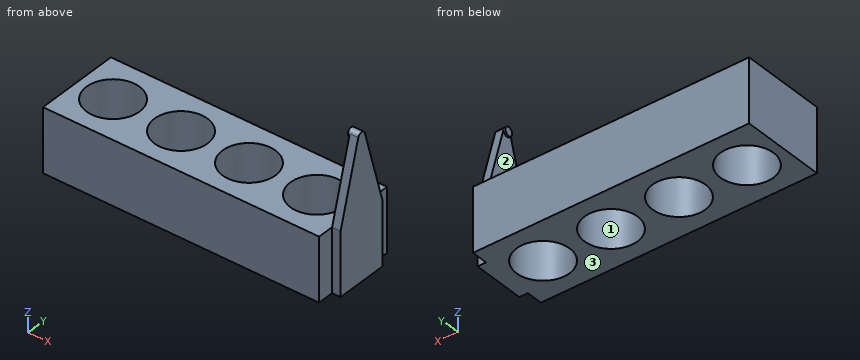
```python
from build123d import *

# Parameters (mm, degrees)
F0_W     = 130
F0_H     = 40
F0_R     = 12.5
F1_DEPTH = 30
F2_W     = 12.3288280059
F2_H     = 30
F3_DEPTH = 4
F4_DEPTH = 4
F6_DEPTH = 0.88206


with BuildPart() as f1:
    # F0 (on Top) → F1 (new body)
    with BuildSketch(Plane.XY):
        Rectangle(F0_W, F0_H)
        with Locations((-48, 0)):
            Circle(F0_R, mode=Mode.SUBTRACT)
        with Locations((-16, 0)):
            Circle(F0_R, mode=Mode.SUBTRACT)
        with Locations((16, 0)):
            Circle(F0_R, mode=Mode.SUBTRACT)
        with Locations((48, 0)):
            Circle(F0_R, mode=Mode.SUBTRACT)
    extrude(amount=F1_DEPTH)

    # F2 (on face) → F3 (join)
    with BuildSketch(Plane.YZ.offset(65)):
        with BuildLine():
            Line((-12.3288280059, 30), (0, 30))
            Line((0, 30), (0, 64))
            ThreePointArc((0, 64), (-1.5961346024, 64.7948633558), (-1.9235602984, 66.5476456688))
            Line((-1.9235602984, 66.5476456688), (-12.3288280059, 30))
        make_face()
        with BuildLine():
            Line((0, 64), (0, 30))
            Line((0, 30), (12.3288280059, 30))
            Line((12.3288280059, 30), (1.9235602984, 66.5476456688))
            ThreePointArc((1.9235602984, 66.5476456688), (1.9807978944, 66.2764773076), (2, 66))
            ThreePointArc((2, 66), (1.4142135624, 64.5857864376), (0, 64))
        make_face()
        with Locations((6.164414003, 15)):
            Rectangle(F2_W, F2_H)
        with Locations((-6.164414003, 15)):
            Rectangle(F2_W, F2_H)
    extrude(amount=F3_DEPTH)

    # F2 (on face) → F4 (join)
    with BuildSketch(Plane.YZ.offset(65)):
        with BuildLine():
            Line((0, 0), (0, 30))
            Line((0, 30), (0, 64))
            ThreePointArc((0, 64), (-1.5961346024, 64.7948633558), (-1.9235602984, 66.5476456688))
            Line((-1.9235602984, 66.5476456688), (-12.3288280059, 30))
            Line((-12.3288280059, 30), (-12.3288280059, 0))
            Line((-12.3288280059, 0), (0, 0))
        make_face()
        with BuildLine():
            Line((0, 64), (0, 30))
            Line((0, 30), (0, 0))
            Line((0, 0), (12.3288280059, 0))
            Line((12.3288280059, 0), (12.3288280059, 30))
            Line((12.3288280059, 30), (1.9235602984, 66.5476456688))
            ThreePointArc((1.9235602984, 66.5476456688), (1.9807978944, 66.2764773076), (2, 66))
            ThreePointArc((2, 66), (1.4142135624, 64.5857864376), (0, 64))
        make_face()
        with BuildLine():
            ThreePointArc((-1.9235602984, 66.5476456688), (-1.5961346024, 64.7948633558), (0, 64))
            ThreePointArc((0, 64), (1.4142135624, 64.5857864376), (2, 66))
            ThreePointArc((2, 66), (1.9807978944, 66.2764773076), (1.9235602984, 66.5476456688))
            ThreePointArc((1.9235602984, 66.5476456688), (0, 68), (-1.9235602984, 66.5476456688))
        make_face()
    extrude(amount=F4_DEPTH)

    # F5 (on face) → F6 (join)
    with BuildSketch(Plane(origin=(65, 0, 0), x_dir=(0, -1, 0), z_dir=(-1, 0, 0))):
        with BuildLine():
            ThreePointArc((-1.9235602984, 66.5476456688), (-0.2764773076, 64.0192021056), (2, 66))
            ThreePointArc((2, 66), (1.9807978944, 66.2764773076), (1.9235602984, 66.5476456688))
            ThreePointArc((1.9235602984, 66.5476456688), (0, 68), (-1.9235602984, 66.5476456688))
        make_face()
    extrude(amount=F6_DEPTH)


solid = f1.part
```
Build history of the part. All positions in model axes, mm. Face numbers are marked on the shaded views. Give positions to 0.01 mm unless a question says otherwise; leave off trailing zeros. Loops run counter-clockwise (first coordinate to the right, second up) from the corner with the lowest first, then second, coordinate; pieces in that order, holes last.
Item 1: Pull direction Z, two halves, no side cores. Call the marked faces 1, 2 and 3: released by +Z, released by -Z, zero draft, split by the parting line, or undercut.
Answers follow:
face 1: zero draft
face 2: undercut
face 3: released by -Z
Item 2: Slice it at C-C, the plane z = 22.5. List the corners of the cut face in (x, y).
Answers follow:
outline: (-65, -20) - (65, -20) - (65, -12.33) - (69, -12.33) - (69, 12.33) - (65, 12.33) - (65, 20) - (-65, 20) - close; hole circle Ø25 at (-48, 0); hole circle Ø25 at (-16, 0); hole circle Ø25 at (16, 0); hole circle Ø25 at (48, 0)
Item 3: Slice it at B-B, the plane x = 58. List the corners of the cut face in (y, z), and give its area (3 significant figures).
Answers follow:
outline: (-20, 0) - (-7.5, 0) - (-7.5, 30) - (-20, 30) - close; (7.5, 0) - (20, 0) - (20, 30) - (7.5, 30) - close
area: 750 mm2
Item 4: Drill centre lines: line 1 (Y direction, x = -48, z = 14); line 2 (Z direction, x = -21, y = -12.5); line 3 (Y direction, x = -37.5, z = 15.5). Where is each one in solid material? Low to high.
Answers follow:
line 1: y = -20 to -12.5, 12.5 to 20
line 2: z = 0 to 30
line 3: y = -20 to -6.78, 6.78 to 20
Item 5: Slice it at A-A, the plane y = 0. List the corners of the cut face in (x, z), and give its area (3 significant figures).
Answers follow:
outline: (-65, 0) - (-60.5, 0) - (-60.5, 30) - (-65, 30) - close; (-35.5, 0) - (-28.5, 0) - (-28.5, 30) - (-35.5, 30) - close; (-3.5, 0) - (3.5, 0) - (3.5, 30) - (-3.5, 30) - close; (28.5, 0) - (35.5, 0) - (35.5, 30) - (28.5, 30) - close; (60.5, 0) - (69, 0) - (69, 68) - (64.12, 68) - (64.12, 64) - (65, 64) - (65, 30) - (60.5, 30) - close
area: 1,180 mm2
Item 6: Slice it at D-D, the plane x = -48. List the corners of the cut face in (y, z), and give its area (3 significant figures).
Answers follow:
outline: (-20, 0) - (-12.5, 0) - (-12.5, 30) - (-20, 30) - close; (12.5, 0) - (20, 0) - (20, 30) - (12.5, 30) - close
area: 450 mm2
Item 7: Flat gauge pins, fed straight in: pin 1 (3 mm diameter, centred on x = 39, y = 11.5, fed in from +Z); pin 2 (1 mm diameter, centred on x = 31, y = 15.5, fed in from -Z); pin 3 (1.2 mm diameter, centred on x = 67, z = 16, fed in from -Y); pin 4 (1.2 mm diameter, centred on x = 67, z = 8, fed in from +Y). Where does each tip first touch, or does it go through?
Answers follow:
pin 1: stops at z = 30
pin 2: stops at z = 0
pin 3: stops at y = -12.33
pin 4: stops at y = 12.33
